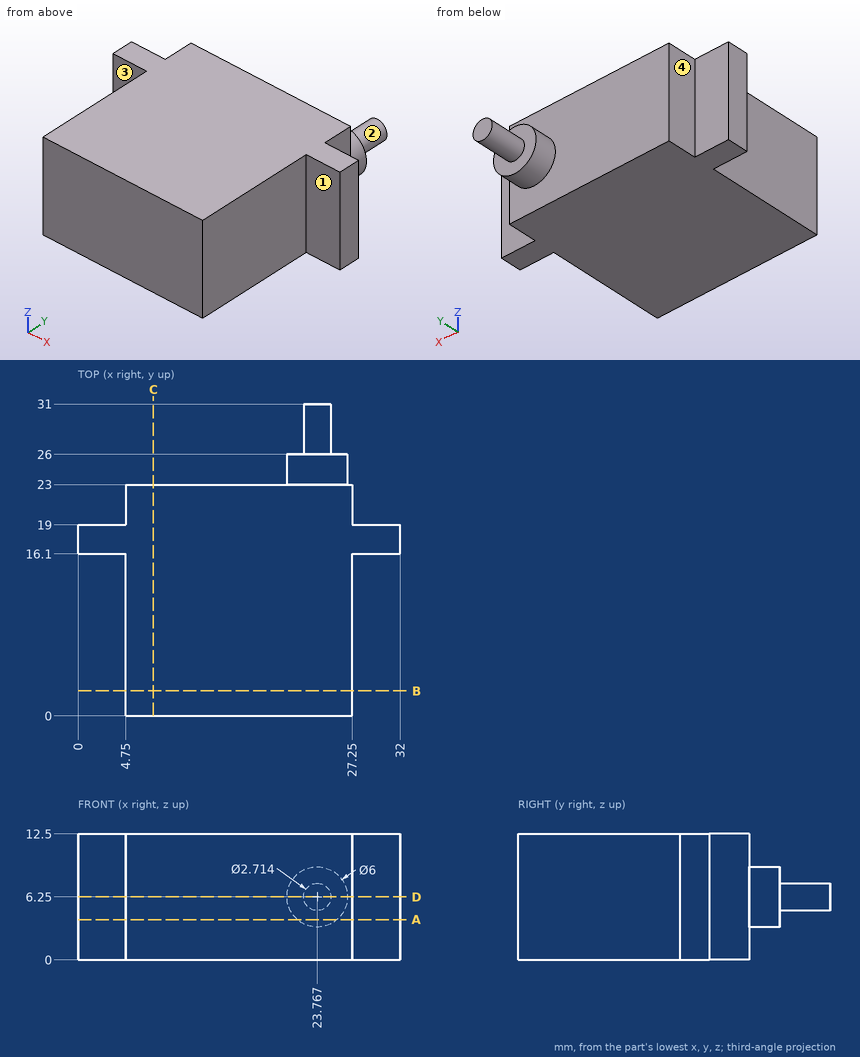
For this review, use the dimensioned drawing (mm, ordinates from the lowest corner) and the shaded views. A direction names the side the tool comes from. Round coordinates to 2 decimals unless told otherwise and drop trailing zeros. Write each loop counter-clockwise with the first axis right and the second up, starting at its lowest first coordinate (ties: lowest second). Pieces come first, ordered by that corner, then holes. Notation, with made-up numbers: (77.25, 30) - (112.25, 30) arc R35 ccw to (112.25, 62) - close; hole circle Ø6 at (33, 13). An arc over 180 degrees is marked (long way). One line per item, written item: value. Start each with the question number.
1. Consider section A-A on z = 4. Write out the cut boundary in (x, y).
2. Clearance check with flat-ended pins moving along their axes: P1, Ø6, axis at x = 13, z = 5, coming from the +Y side; P2, Ø4, axis at y = 12, z = 5.5, coming from the -X side; P3, Ø2, axis at y = 21.5, z = 5.5, coming from the +X side. State where each tip first meets the part, or that it passes through.
3. Consider section B-B on y = 2.5. Write out the cut boundary in (x, z), and give its area (3 significant figures).
4. Consider section D-D on z = 6.25. Write out the cut boundary in (x, y), and give its area (3 significant figures).
5. To check wall thickness, follow L1, parallel to Y at x = 6, z = 3.5; L2, parallel to Y at x = 2, z = 1.5; L3, parallel to X at y = 15.5, z = 1.75. State the ranges of each line that lie inside material, in increasing order. Write a range as from..to.
6. Consider section C-C on x = 7.5. Write out the cut boundary in (y, z).
7. Machinability: for the marked faces 1, 2, 3 and 4, which of the approach directions +Z, -Z, +X, -X, +Y, -Y give a long, thin tool a straight path to every point of the face, cutting with its end or side? Answer none if there is none.
Checks:
1. outline: (0, 16.1) - (4.75, 16.1) - (4.75, 0) - (27.25, 0) - (27.25, 16.1) - (32, 16.1) - (32, 19) - (27.25, 19) - (27.25, 23) - (25.75, 23) - (25.75, 26) - (21.78, 26) - (21.78, 23) - (4.75, 23) - (4.75, 19) - (0, 19) - close
2. P1: stops at y = 23
2. P2: stops at x = 4.75
2. P3: stops at x = 27.25
3. outline: (4.75, 0) - (27.25, 0) - (27.25, 12.5) - (4.75, 12.5) - close
3. area: 281 mm^2
4. outline: (0, 16.1) - (4.75, 16.1) - (4.75, 0) - (27.25, 0) - (27.25, 16.1) - (32, 16.1) - (32, 19) - (27.25, 19) - (27.25, 23) - (26.77, 23) - (26.77, 26) - (25.12, 26) - (25.12, 31) - (22.41, 31) - (22.41, 26) - (20.77, 26) - (20.77, 23) - (4.75, 23) - (4.75, 19) - (0, 19) - close
4. area: 577 mm^2
5. L1: y = 0..23
5. L2: y = 16.1..19
5. L3: x = 4.75..27.25
6. outline: (0, 0) - (23, 0) - (23, 12.5) - (0, 12.5) - close
7. face 1: +Z, -Z, +X, -Y
7. face 2: +Y
7. face 3: +Z, -Z, -X, -Y
7. face 4: +Z, -Z, -X, +Y
